The model under review builds one solid part; all positions refer to its coordinate system, in mm. A direction names the side the tool comes from. Round coordinates to 2 decimals unless told otherwise and drop trailing zeros. Loops run counter-clockwise (first coordinate to the right, second up) from the corner with the lowest first, then second, coordinate; pieces in that order, holes last. Notation, with made-up numbers: M 86.5,22 L 118.5,22 A21 ccw 118.5,49 Z; hole C -9.5,-35 d2. An arc over 180 degrees is marked long. Answer as a JSON object with one key per item and string values. Group by question number.
Item 1: Insertion check: P1, Ø6.5, axis at y = 50, z = 75.5, coming from the -X side; P2, Ø3, axis at x = 76, y = 19.5, coming from the +Z side; P3, Ø1.5, axis at y = 4.5, z = 59, coming from the -X side; P4, Ø12, axis at x = 79, z = 17, coming from the +Y side. Each pin has a flat end and moves straight along its axis. Give the tip position at first contact, or say it passes through.
Item 2: Consider section A-A (y = 65). State how many separate pieces and enclosed holes the cut face has, and give its area (3 significant figures).
Item 3: To check wall thickness, follow line 1 (Z direction, x = 31, y = 58.5); line 2 (Z direction, x = 62, y = 22); line 3 (X direction, y = 47, z = 5.5). State the ranges of each line that lie inside material, in increasing order.
Item 4: Consider section D-D (x = 90). Give the boundary of the cut face in (y, z), and give its area (4 significant figures).
Item 5: Consider section B-B (z = 14). Give the boundary of the cut face in (x, y).
Item 6: The part is to be moulded in two halves that separate along Z. For faces 4 (the face through (68.859, 14.755, 65.361)), 5 (the face through (98, 1, 5)), 6 (the face through (60.4, 49.3, 0)), say which applies: +Z half, -Z half, draft (parallel to the pull), parting line (faces both ways), or undercut.
Item 7: Tool access review of faces 1 (the face through (33.549, 20.751, 17.115)), 2 (the face through (36, 84, 32)), 3 (the face through (66.451, 5.251, 62.384)): name each direction out of +Z, -Z, +X, -X, +Y, -Y from which nothing blocks a thin tool from reaching the whole face with its end or side.
Item 8: Consider section C-C (x = 47). Give the boundary of the cut face in (y, z), and give its area (3 significant figures).
```python
from build123d import *

# Parameters (mm, degrees)
SKETCH1_W                  = 79.99984
SKETCH1_H                  = 90.999818
BOSS_EXTRUDE1_DEPTH        = 67.7498645
BOSS_EXTRUDE2_DEPTH        = 32.2499355
CUT_EXTRUDE1_DEPTH         = 29.99994
SKETCH4_W                  = 29.99994
SKETCH4_H                  = 90.999818
CUT_EXTRUDE2_DEPTH         = 13.999972
SKETCH5_W                  = 69.99986
SKETCH5_H                  = 90.999818
CUT_EXTRUDE3_DEPTH         = 29.99994
SKETCH6_W                  = 39.99992
SKETCH6_H                  = 74.99985
BOSS_EXTRUDE3_DEPTH        = 2.2499955
SKETCH7_W                  = 19.99996
SKETCH7_H                  = 69.99986
CUT_EXTRUDE4_DEPTH         = 29.99994
SKETCH8_W                  = 39.99992
SKETCH8_H                  = 69.99986
CUT_EXTRUDE5_DEPTH         = 34.99993
SKETCH9_W                  = 46.999906
SKETCH9_H                  = 81.999836
SKETCH9_W_2                = 39.99992
SKETCH9_H_2                = 74.99985
CUT_EXTRUDE6_DEPTH         = 2.2499955
BOSS_EXTRUDE4_DEPTH        = 8.999982
F_10_CLEARANCE_HOLE1_D     = 4.99999
F_10_CLEARANCE_HOLE1_DEPTH = 6.999986
F_10_CLEARANCE_HOLE2_D     = 4.99999
F_10_CLEARANCE_HOLE2_DEPTH = 6.999986
FILLET1_R                  = 4.99999
FILLET2_R                  = 7.499985
FILLET3_R                  = 10.999978


with BuildPart() as part:
    # Sketch1 → Boss-Extrude1 (new body)
    with BuildSketch(Plane(origin=(99.9998, 0, 0), x_dir=(0, 0, -1), z_dir=(1, 0, 0))):
        with Locations((-39.99992, 45.499909)):
            Rectangle(SKETCH1_W, SKETCH1_H)
    extrude(amount=-BOSS_EXTRUDE1_DEPTH)

    # Sketch2 → Boss-Extrude2 (add)
    with BuildSketch(Plane.ZY.offset(-32.2499355)):
        Polygon((0, 90.999818), (23.999952, 90.999818), (23.999952, 8.999982), (70.999858, 8.999982), (70.999858, 90.999818), (79.99984, 90.999818), (79.99984, 0), (0, 0), align=None)
    extrude(amount=BOSS_EXTRUDE2_DEPTH)

    # Sketch3 → Cut-Extrude1 (cut)
    with BuildSketch(Plane.ZY):
        Polygon((70.999858, 8.999982), (23.999952, 8.999982), (23.999952, 0), (79.99984, 0), (79.99984, 90.999818), (70.999858, 90.999818), align=None)
    extrude(amount=-CUT_EXTRUDE1_DEPTH, mode=Mode.SUBTRACT)

    # Sketch4 → Cut-Extrude2 (cut)
    with BuildSketch(Plane.XY.offset(23.999952)):
        with Locations((14.99997, 45.499909)):
            Rectangle(SKETCH4_W, SKETCH4_H)
    extrude(amount=-CUT_EXTRUDE2_DEPTH, mode=Mode.SUBTRACT)

    # Sketch5 → Cut-Extrude3 (cut)
    with BuildSketch(Plane(origin=(99.9998, 0, 0), x_dir=(0, 0, -1), z_dir=(1, 0, 0))):
        with Locations((-44.99991, 45.499909)):
            Rectangle(SKETCH5_W, SKETCH5_H)
    extrude(amount=-CUT_EXTRUDE3_DEPTH, mode=Mode.SUBTRACT)

    # Sketch6 → Boss-Extrude3 (add)
    with BuildSketch(Plane.ZY.offset(-32.2499355)):
        with Locations((47.499905, 49.9999)):
            Rectangle(SKETCH6_W, SKETCH6_H)
    extrude(amount=BOSS_EXTRUDE3_DEPTH)

    # Sketch7 → Cut-Extrude4 (cut)
    with BuildSketch(Plane(origin=(0, 0, 0), x_dir=(-1, 0, 0), z_dir=(0, 0, -1))):
        with Locations((-49.9999, 49.9999)):
            Rectangle(SKETCH7_W, SKETCH7_H)
    extrude(amount=-CUT_EXTRUDE4_DEPTH, mode=Mode.SUBTRACT)

    # Sketch8 → Cut-Extrude5 (cut)
    with BuildSketch(Plane(origin=(0, 0, 29.99994), x_dir=(-1, 0, 0), z_dir=(0, 0, -1))):
        with Locations((-49.9999, 49.9999)):
            Rectangle(SKETCH8_W, SKETCH8_H)
    extrude(amount=-CUT_EXTRUDE5_DEPTH, mode=Mode.SUBTRACT)

    # Sketch9 → Cut-Extrude6 (cut)
    with BuildSketch(Plane(origin=(69.99986, 0, 0), x_dir=(0, 0, -1), z_dir=(1, 0, 0))):
        with Locations((-47.499905, 49.9999)):
            Rectangle(SKETCH9_W, SKETCH9_H)
        with Locations((-47.499905, 49.9999)):
            Rectangle(SKETCH9_W_2, SKETCH9_H_2, mode=Mode.SUBTRACT)
    extrude(amount=-CUT_EXTRUDE6_DEPTH, mode=Mode.SUBTRACT)

    # Sketch10 → Boss-Extrude4 (add)
    with BuildSketch(Plane(origin=(0, 90.999818, 0), x_dir=(-1, 0, 0), z_dir=(0, 1, 0))):
        Polygon((-29.99994, 9.99998), (0, 9.99998), (0, 0), (-99.9998, 0), (-99.9998, 9.99998), (-69.99986, 9.99998), (-69.99986, 79.99984), (-29.99994, 79.99984), align=None)
    extrude(amount=BOSS_EXTRUDE4_DEPTH)

    # #10 Clearance Hole1
    with Locations(Plane.ZY.offset(-29.99994)):
        with Locations((19.499961, 79.99984), (59.99988, 95.499809), (19.499961, 49.9999), (34.99993, 4.499991), (75.499849, 19.99996), (75.499849, 49.9999), (59.99988, 4.499991), (19.499961, 19.99996), (75.499849, 79.99984), (34.99993, 95.499809)):
            Hole(F_10_CLEARANCE_HOLE1_D / 2, depth=F_10_CLEARANCE_HOLE1_DEPTH)

    # #10 Clearance Hole2
    with Locations(Plane(origin=(69.99986, 0, 0), x_dir=(0, 0, -1), z_dir=(1, 0, 0))):
        with Locations((-59.99988, 4.499991), (-75.499849, 49.9999), (-59.99988, 95.499809), (-19.499961, 79.99984), (-19.499961, 19.99996), (-34.99993, 4.499991), (-19.499961, 49.9999), (-34.99993, 95.499809), (-75.499849, 79.99984), (-75.499849, 19.99996)):
            Hole(F_10_CLEARANCE_HOLE2_D / 2, depth=F_10_CLEARANCE_HOLE2_DEPTH)

    # Fillet1
    fillet1_edges = [part.edges().sort_by_distance(p)[0] for p in [
        (59.99988, 14.99997, 14.99997),
        (59.99988, 84.99983, 14.99997),
        (39.99992, 84.99983, 14.99997),
        (39.99992, 14.99997, 14.99997),
        (64.99987, 84.99983, 29.99994),
        (64.99987, 14.99997, 29.99994),
        (49.9999, 14.99997, 64.99987),
        (49.9999, 84.99983, 64.99987),
        (34.99993, 14.99997, 29.99994),
        (34.99993, 84.99983, 29.99994),
        (99.9998, 99.9998, 4.99999),
        (0, 99.9998, 4.99999),
        (0, 0, 4.99999),
        (99.9998, 0, 4.99999),
    ]]
    fillet(fillet1_edges, radius=FILLET1_R)

    # Fillet2
    fillet2_edges = [part.edges().sort_by_distance(p)[0] for p in [
        (68.87486225, 87.499825, 67.499865),
        (68.87486225, 87.499825, 27.499945),
        (68.87486225, 12.499975, 27.499945),
        (68.87486225, 12.499975, 67.499865),
        (31.12493775, 87.499825, 27.499945),
        (31.12493775, 12.499975, 27.499945),
        (31.12493775, 12.499975, 67.499865),
        (31.12493775, 87.499825, 67.499865),
    ]]
    fillet(fillet2_edges, radius=FILLET2_R)

    # Fillet3
    fillet3_edges = [part.edges().sort_by_distance(p)[0] for p in [
        (68.87486225, 8.999982, 70.999858),
        (68.87486225, 90.999818, 70.999858),
        (68.87486225, 90.999818, 23.999952),
        (68.87486225, 8.999982, 23.999952),
        (31.12493775, 8.999982, 23.999952),
        (31.12493775, 8.999982, 70.999858),
        (31.12493775, 90.999818, 70.999858),
        (31.12493775, 90.999818, 23.999952),
    ]]
    fillet(fillet3_edges, radius=FILLET3_R)


solid = part.part
```
Geometry results:
{
 "1": {"P1": "stops at x = 30", "P2": "stops at z = 10", "P3": "stops at x = 37", "P4": "passes through"},
 "2": {"separate pieces": "3", "enclosed holes": "0", "area": "1,770 mm^2"},
 "3": {"line 1": "z = 0 to 24, 27.5 to 30, 65 to 67.5, 71 to 80", "line 2": "z = 0 to 30, 65 to 80", "line 3": "x = 0 to 40, 60 to 100"},
 "4": {"outline": "M 0,0 L 100,0 L 100,10 L 0,10 Z", "area": "1,000 mm^2"},
 "5": {"outline": "M 30,0 L 70,0 L 70,100 L 30,100 Z; hole M 40,20 A5 ccw 45,15 L 55,15 A5 ccw 60,20 L 60,80 A5 ccw 55,85 L 45,85 A5 ccw 40,80 Z"},
 "6": {"face 4": "undercut", "face 5": "draft", "face 6": "-Z half"},
 "7": {"face 1": "-X", "face 2": "+X, -X", "face 3": "+X"},
 "8": {"outline": "M 0,0 L 15,0 L 15,60 A5 cw 20,65 L 80,65 A5 cw 85,60 L 85,0 L 100,0 L 100,80 L 0,80 Z", "area": "3,460 mm^2"}
}
